Source: three-view drawing plus pictorial views. Frame: mm from the lowest corner of the part. Give positions to 0.01 mm unless a question says otherwise; leave off trailing zeros. Write each loop counter-clockwise with the first axis right and the second up, starting at its lowest first coordinate (ties: lowest second). Pieces come first, ordered by that corner, then holes.
Q1. Cut plane A-A on y = 175. Return the cut outline in (x, z), plus the area to 3 significant figures.
Q2. Cut plane D-D on y = 25. Return the cut outline in (x, z), plus the area to 3 significant figures.
Q3. Line query: L1, parallel to Y at x = 50, z = 2.75; L2, parallel to Y at x = 47.5, z = 1. Output: solid intervals per line, ascending.
Q4. Cut plane C-C on z = 6.5. Return the cut outline in (x, y), plus the area to 3 significant figures.
Q5. Cut plane B-B on x = 50. Return the cut outline in (y, z).
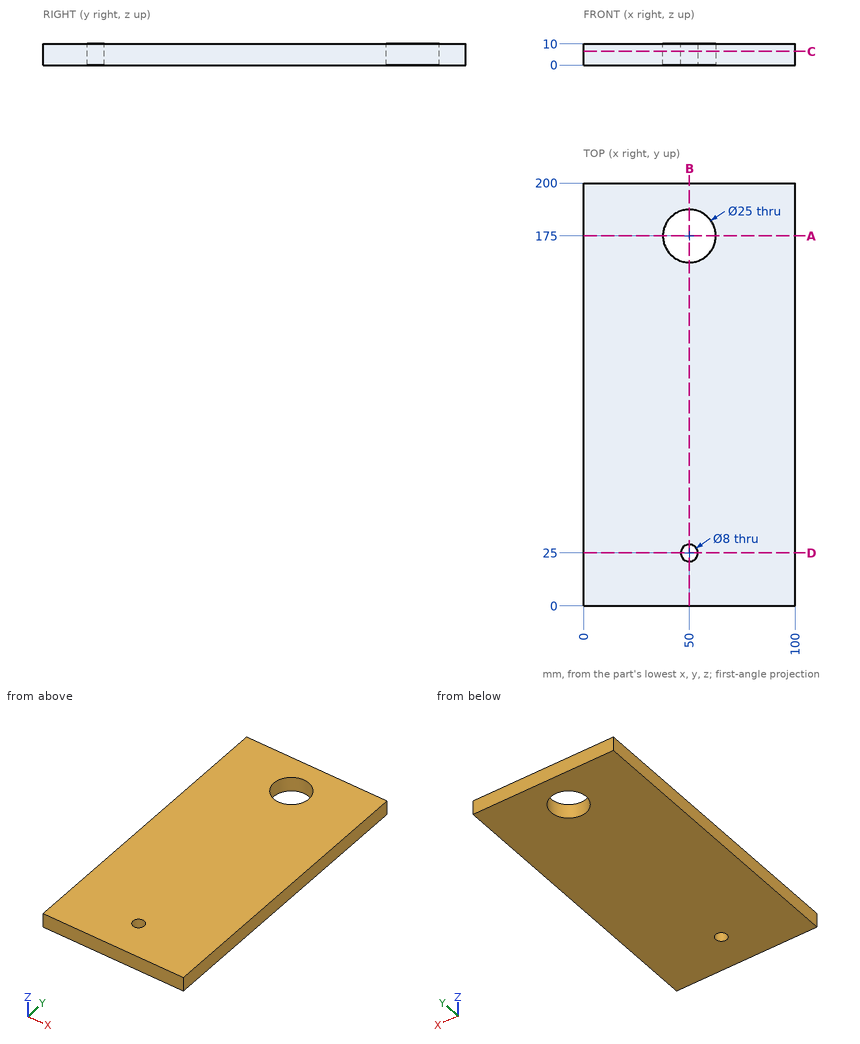
Data:
1. outline: (0, 0) - (37.5, 0) - (37.5, 10) - (0, 10) - close; (62.5, 0) - (100, 0) - (100, 10) - (62.5, 10) - close
1. area: 750 mm2
2. outline: (0, 0) - (46, 0) - (46, 10) - (0, 10) - close; (54, 0) - (100, 0) - (100, 10) - (54, 10) - close
2. area: 920 mm2
3. L1: y = 0 to 21, 29 to 162.5, 187.5 to 200
3. L2: y = 0 to 21.88, 28.12 to 162.75, 187.25 to 200
4. outline: (0, 0) - (100, 0) - (100, 200) - (0, 200) - close; hole circle Ø25 at (50, 175); hole circle Ø8 at (50, 25)
4. area: 19,500 mm2
5. outline: (0, 0) - (21, 0) - (21, 10) - (0, 10) - close; (29, 0) - (162.5, 0) - (162.5, 10) - (29, 10) - close; (187.5, 0) - (200, 0) - (200, 10) - (187.5, 10) - close
